Input: dimensioned drawing with shaded views. Units: mm. Origin: part minimum x, y, z. A direction names the side the tool comes from. Round coordinates to 2 decimals unless told otherwise and drop trailing zeros. Loops run counter-clockwise (first coordinate to the right, second up) from the corner with the lowest first, then second, coordinate; pieces in that order, holes last.
Item 1: Section query C-C on x = 7.25. Return loops of the section in (y, z) (3 decimals).
Item 2: Section query D-D on x = 1.5. Return loops of the section in (y, z) (3 decimals).
Item 3: First-contact query: P1, Ø4, axis at y = 11.025, z = 18.775, coming from the +X side; P2, Ø2, axis at x = 3.5, z = 11.5, coming from the +Y side (3 decimals); P3, Ø1, axis at y = 8.5, z = 16.5, coming from the -X side. Flat tips, straight axial feed; report the tip coordinate or a pass-through.
Item 4: Section query B-B on y = 17.75. Return loops of the section in (x, z), then the cut area to 3 significant figures.
Item 5: Access query for the marked faces 1 and 2. Directions: +Z, -Z, +X, -X, +Y, -Y. A direction counts if a zero-diameter tool reaches every point of the face in a straight line with its end or side. Return the directions, or none.
Item 6: Section query A-A on z = 7.5. Return loops of the section in (x, y), then the cut area to 3 significant figures.
Item 7: Ray query, L1, parallel to X at y = 17, z = 19.75; L2, parallel to Y at x = 3, z = 9.75; L3, parallel to Z at x = 7.75, y = 12. Return the intervals inside material, ascending.
Item 8: Pull-direction query (Y, two-part tool) for the marked faces 3, 4 and 5; classes: released by +Y, released by -Y, zero draft, split by the parting line, or undercut.
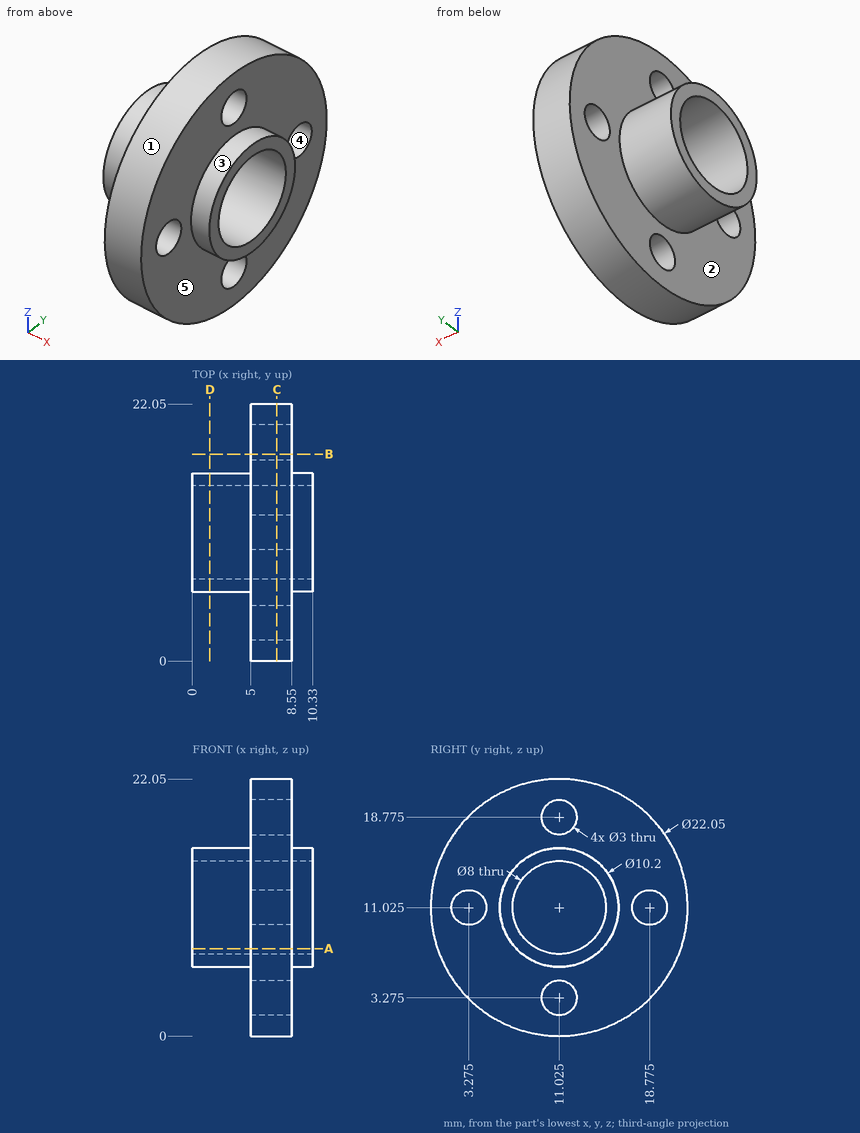
Data:
1. outline: circle Ø22.05 at (11.025, 11.025); hole circle Ø3 at (3.275, 11.025); hole circle Ø8 at (11.025, 11.025); hole circle Ø3 at (11.025, 3.275); hole circle Ø3 at (11.025, 18.775); hole circle Ø3 at (18.775, 11.025)
2. outline: circle Ø10.2 at (11.025, 11.025); hole circle Ø8 at (11.025, 11.025)
3. P1: stops at x = 8.55
3. P2: stops at y = 16.125
3. P3: stops at x = 5
4. outline: (5, 2.29) - (8.55, 2.29) - (8.55, 9.93) - (5, 9.93) - close; (5, 12.12) - (8.55, 12.12) - (8.55, 19.76) - (5, 19.76) - close
4. area: 54.3 mm2
5. face 1: +X, -X
5. face 2: -X
6. outline: (0, 7.34) - (5, 7.34) - (5, 0.58) - (8.55, 0.58) - (8.55, 7.34) - (10.33, 7.34) - (10.33, 9.13) - (0, 9.13) - close; (0, 12.92) - (10.33, 12.92) - (10.33, 14.71) - (8.55, 14.71) - (8.55, 21.47) - (5, 21.47) - (5, 14.71) - (0, 14.71) - close
6. area: 85.1 mm2
7. L1: x = 5 to 8.55
7. L2: y = 6.09 to 7.23, 14.82 to 15.96
7. L3: z = 0.04 to 2.14, 4.41 to 7.15, 14.9 to 17.64, 19.91 to 22.01
8. face 3: split by the parting line
8. face 4: undercut
8. face 5: zero draft
